Check sheet for the modelled part. Datum: model origin and axes. Units: mm. Face numbers are marked on the shaded views. Coordinates: 2 decimals unless noted, no trailing zeros. Write each loop counter-clockwise with the first axis right and the second up, starting at its lowest first coordinate (ties: lowest second). Pieces come first, ordered by that corner, then holes. Notation, with made-up numbers: (79, 84.5) - (87, 84.5) arc R14 cw to (87, 93.5) - close; hole circle Ø4 at (-25.5, 61.25). An arc over 180 degrees is marked (long way). Write each question's results on one line, items separated by ' | '.
from build123d import *

# Parameters (mm, degrees)
BOSS_EXTRUDE1_DEPTH = 12.7
CUT_EXTRUDE2_DEPTH  = 199.932436772
CUT_EXTRUDE1_DEPTH  = 104.050150898
CUT_EXTRUDE3_DEPTH  = 63.5
CHAMFER1_SIZE       = 1.5875
FILLET1_R           = 0.762
FILLET2_R           = 1.27


# Some blends are built 0.0001 mm under size
with BuildPart() as part:
    # Sketch1 → Boss-Extrude1 (new body)
    with BuildSketch(Plane(origin=(0, 0, 0), x_dir=(1, 0, 0), z_dir=(0, 1, 0))):
        with BuildLine():
            Line((-99.06, -12.7), (99.06, -12.7))
            Line((99.06, -12.7), (99.06, -11.1125))
            Line((99.06, -11.1125), (80.01, -11.1125))
            ThreePointArc((80.01, -11.1125), (75.519871939, -9.252628061), (73.66, -4.7625))
            Line((73.66, -4.7625), (73.66, 4.7625))
            ThreePointArc((73.66, 4.7625), (75.519871939, 9.252628061), (80.01, 11.1125))
            Line((80.01, 11.1125), (99.06, 11.1125))
            Line((99.06, 11.1125), (99.06, 12.7))
            Line((99.06, 12.7), (-99.06, 12.7))
            Line((-99.06, 12.7), (-99.06, 11.1125))
            Line((-99.06, 11.1125), (-80.01, 11.1125))
            ThreePointArc((-80.01, 11.1125), (-75.519871939, 9.252628061), (-73.66, 4.7625))
            Line((-73.66, 4.7625), (-73.66, -4.7625))
            ThreePointArc((-73.66, -4.7625), (-75.519871939, -9.252628061), (-80.01, -11.1125))
            Line((-80.01, -11.1125), (-99.06, -11.1125))
            Line((-99.06, -11.1125), (-99.06, -12.7))
        make_face()
    extrude(amount=BOSS_EXTRUDE1_DEPTH)

    # Sketch3 → Cut-Extrude2 (cut, through all)
    with BuildSketch(Plane.ZY.offset(99.06)):
        Polygon((11.1125, 12.7), (4.7625, 12.7), (-4.7625, 12.7), (-11.1125, 12.7), (-9.525, 6.35), (9.525, 6.35), align=None)
    extrude(amount=-CUT_EXTRUDE2_DEPTH, mode=Mode.SUBTRACT)

    # Sketch2 → Cut-Extrude1 (cut, through all)
    with BuildSketch(Plane.XY.offset(12.7)):
        Polygon((73.66, 12.7), (-73.66, 12.7), (-67.31, 6.35), (67.31, 6.35), align=None)
        with BuildLine():
            Line((97.263948776, 4.553948776), (92.71, 0))
            Line((92.71, 0), (99.06, 0))
            Line((99.06, 0), (99.06, 12.7))
            Line((99.06, 12.7), (92.71, 12.7))
            Line((92.71, 12.7), (97.263948776, 8.146051224))
            ThreePointArc((97.263948776, 8.146051224), (98.007897552, 6.35), (97.263948776, 4.553948776))
        make_face()
        with BuildLine():
            ThreePointArc((-97.263948776, 4.553948776), (-98.007897552, 6.35), (-97.263948776, 8.146051224))
            Line((-97.263948776, 8.146051224), (-92.71, 12.7))
            Line((-92.71, 12.7), (-99.06, 12.7))
            Line((-99.06, 12.7), (-99.06, 0))
            Line((-99.06, 0), (-92.71, 0))
            Line((-92.71, 0), (-97.263948776, 4.553948776))
        make_face()
    extrude(amount=-CUT_EXTRUDE1_DEPTH, mode=Mode.SUBTRACT)

    # Sketch4 → Revolve1 (revolve)
    with BuildSketch(Plane.ZY.offset(90.17)):
        with BuildLine():
            Line((12.7, 6.35), (12.7, 11.43))
            ThreePointArc((12.7, 11.43), (13.881381744, 9.01113492), (14.2875, 6.35))
            Line((14.2875, 6.35), (12.7, 6.35))
        make_face()
    revolve1 = revolve(axis=Axis((-90.17, 6.35, 0), (0, 0, 1)))

    # Mirror1: Revolve1 across plane
    add(revolve1.mirror(Plane.XY))

    # Sketch5 → Revolve2 (revolve)
    with BuildSketch(Plane(origin=(90.17, 0, 0), x_dir=(0, 0, -1), z_dir=(1, 0, 0))):
        with BuildLine():
            Line((11.1125, 6.35), (11.1125, 11.43))
            ThreePointArc((11.1125, 11.43), (9.931118256, 9.01113492), (9.525, 6.35))
            Line((9.525, 6.35), (11.1125, 6.35))
        make_face()
    revolve2 = revolve(axis=Axis((90.17, 6.35, 0), (0, 0, -1)))

    # Mirror2: Revolve2 across plane
    add(revolve2.mirror(Plane.XY))

    # Sketch6 → Cut-Extrude3 (cut, symmetric)
    with BuildSketch(Plane(origin=(0, 0, 0), x_dir=(0, 0, -1), z_dir=(1, 0, 0))):
        Polygon((-12.7, 0), (-11.1125, 0), (-12.7, 1.5875), align=None)
        Polygon((11.1125, 0), (12.7, 1.5875), (12.7, 0), align=None)
    extrude(amount=CUT_EXTRUDE3_DEPTH, both=True, mode=Mode.SUBTRACT)

    # Chamfer1
    chamfer1_edges = [part.edges().sort_by_distance(p)[0] for p in [
        (63.5, 0, 11.90625),
        (63.5, 0, -11.90625),
        (-63.5, 0, -11.90625),
        (-63.5, 0, 11.90625),
    ]]
    chamfer(chamfer1_edges, length=CHAMFER1_SIZE - 0.0001)  # a hair under: the kernel refuses the full size

    # Fillet1
    fillet1_edges = [part.edges().sort_by_distance(p)[0] for p in [
        (-98.007897552, 6.35, 12.7),
        (-92.71, 12.7, -11.90625),
        (-94.986974388, 10.423025612, -11.1125),
        (-94.986974388, 10.423025612, -12.7),
        (-94.986974388, 10.423025612, 11.1125),
        (-92.71, 12.7, 11.90625),
        (-94.986974388, 2.276974388, 12.7),
        (-98.007897552, 6.35, -11.1125),
        (-98.007897552, 6.35, 11.1125),
        (-94.986974388, 2.276974388, -11.1125),
        (-94.986974388, 2.276974388, 11.1125),
        (-98.007897552, 6.35, -12.7),
        (-94.986974388, 2.276974388, -12.7),
        (-94.986974388, 10.423025612, 12.7),
        (98.007897552, 6.35, 12.7),
        (92.71, 12.7, 11.90625),
        (92.71, 12.7, -11.90625),
        (94.986974388, 10.423025612, 12.7),
        (94.986974388, 2.276974388, 11.1125),
        (94.986974388, 2.276974388, -11.1125),
        (94.986974388, 2.276974388, -12.7),
        (98.007897552, 6.35, 11.1125),
        (94.986974388, 10.423025612, 11.1125),
        (94.986974388, 10.423025612, -11.1125),
        (98.007897552, 6.35, -12.7),
        (94.986974388, 10.423025612, -12.7),
        (94.986974388, 2.276974388, 12.7),
        (98.007897552, 6.35, -11.1125),
    ]]
    fillet(fillet1_edges, radius=FILLET1_R)

    # Fillet2
    # the kernel refuses this fillet: 1.27 mm, written as the material it takes off along each edge
    with BuildSketch(Plane(origin=(-75.90506403, 14.94506403, -12.7), x_dir=(-0.7071067811865446, -0.7071067811865505, 0), z_dir=(0.7071067811865506, -0.7071067811865446, 0))) as fillet2_piece_1_section:
        with BuildLine():
            CenterArc((FILLET2_R, -FILLET2_R), FILLET2_R, 90, 90)
            Line((0, -FILLET2_R), (0, 0))
            Line((0, 0), (FILLET2_R, 0))
        make_face()
    fillet2_piece_1 = extrude(amount=15.330256121, mode=Mode.PRIVATE)
    fillet2_piece_1 = split(fillet2_piece_1, bisect_by=Plane(origin=(-71.905795305, 6.35, -12.408746665), z_dir=(0, 1, 0)), keep=Keep.TOP, mode=Mode.PRIVATE)
    add(fillet2_piece_1, mode=Mode.SUBTRACT)
    with BuildSketch(Plane(origin=(-65.450815483, 4.490815483, -9.060203871), x_dir=(0.1230914909792504, -0.12309149097924957, -0.9847319278346824), z_dir=(-0.696310623822809, 0.6963106238228031, -0.17407765595558086))) as fillet2_piece_2_section:
        with BuildLine():
            CenterArc((FILLET2_R * 0.840960781889, FILLET2_R), FILLET2_R, 189.874961398, 80.125038602)
            Line((-FILLET2_R * 0.144223584254, FILLET2_R * 0.828501414858), (0, 0))
            Line((0, 0), (FILLET2_R * 0.840960781889, 0))
        make_face()
    fillet2_piece_2 = extrude(amount=14.459594166, mode=Mode.PRIVATE)
    fillet2_piece_2 = split(fillet2_piece_2, bisect_by=Plane(origin=(-71.646234354, 6.35, -10.770930609), z_dir=(0, 1, 0)), keep=Keep.TOP, mode=Mode.PRIVATE)
    add(fillet2_piece_2, mode=Mode.SUBTRACT)
    with BuildSketch(Plane(origin=(-75.519184517, 14.559184517, 11.577296129), x_dir=(-0.7177405625652845, -0.6755205294731655, -0.1688801323683837), z_dir=(0.69631062382278, -0.6963106238227741, -0.17407765595581334))) as fillet2_piece_3_section:
        with BuildLine():
            CenterArc((FILLET2_R * 0.840960781889, -FILLET2_R), FILLET2_R, 90, 80.125038602)
            Line((-FILLET2_R * 0.144223584254, -FILLET2_R * 0.828501414857), (0, 0))
            Line((0, 0), (FILLET2_R * 0.840960781889, 0))
        make_face()
    fillet2_piece_3 = extrude(amount=14.459594166, mode=Mode.PRIVATE)
    fillet2_piece_3 = split(fillet2_piece_3, bisect_by=Plane(origin=(-71.646234354, 6.35, 10.770930609), z_dir=(0, 1, 0)), keep=Keep.TOP, mode=Mode.PRIVATE)
    add(fillet2_piece_3, mode=Mode.SUBTRACT)
    with BuildSketch(Plane(origin=(-75.90506403, 14.94506403, 12.7), x_dir=(-0.7071067811865445, -0.7071067811865505, 0), z_dir=(0.7071067811865506, -0.7071067811865446, 0))) as fillet2_piece_4_section:
        with BuildLine():
            CenterArc((FILLET2_R, FILLET2_R), FILLET2_R, 180, 90)
            Line((0, FILLET2_R), (0, 0))
            Line((0, 0), (FILLET2_R, 0))
        make_face()
    fillet2_piece_4 = extrude(amount=15.330256121, mode=Mode.PRIVATE)
    fillet2_piece_4 = split(fillet2_piece_4, bisect_by=Plane(origin=(-71.905795305, 6.35, 12.408746665), z_dir=(0, 1, 0)), keep=Keep.TOP, mode=Mode.PRIVATE)
    add(fillet2_piece_4, mode=Mode.SUBTRACT)
    with BuildSketch(Plane(origin=(65.06493597, 4.10493597, -12.7), x_dir=(0.7071067811865445, -0.7071067811865506, 0), z_dir=(0.7071067811865506, 0.7071067811865445, 0))) as fillet2_piece_5_section:
        with BuildLine():
            CenterArc((FILLET2_R, -FILLET2_R), FILLET2_R, 90, 90)
            Line((0, -FILLET2_R), (0, 0))
            Line((0, 0), (FILLET2_R, 0))
        make_face()
    fillet2_piece_5 = extrude(amount=15.330256121, mode=Mode.PRIVATE)
    fillet2_piece_5 = split(fillet2_piece_5, bisect_by=Plane(origin=(71.905795305, 6.35, -12.408746665), z_dir=(0, 1, 0)), keep=Keep.TOP, mode=Mode.PRIVATE)
    add(fillet2_piece_5, mode=Mode.SUBTRACT)
    with BuildSketch(Plane(origin=(75.519184517, 14.559184517, -11.577296129), x_dir=(-0.12309149097927001, -0.12309149097926336, -0.9847319278346782), z_dir=(-0.6963106238228061, -0.6963106238228001, 0.17407765595560445))) as fillet2_piece_6_section:
        with BuildLine():
            CenterArc((FILLET2_R * 0.840960781889, FILLET2_R), FILLET2_R, 189.874961398, 80.125038602)
            Line((-FILLET2_R * 0.144223584254, FILLET2_R * 0.828501414858), (0, 0))
            Line((0, 0), (FILLET2_R * 0.84096078189, 0))
        make_face()
    fillet2_piece_6 = extrude(amount=14.459594166, mode=Mode.PRIVATE)
    fillet2_piece_6 = split(fillet2_piece_6, bisect_by=Plane(origin=(71.646234354, 6.35, -10.770930609), z_dir=(0, 1, 0)), keep=Keep.TOP, mode=Mode.PRIVATE)
    add(fillet2_piece_6, mode=Mode.SUBTRACT)
    with BuildSketch(Plane(origin=(65.06493597, 4.10493597, 12.7), x_dir=(0.7071067811865445, -0.7071067811865507, 0), z_dir=(0.7071067811865506, 0.7071067811865445, 0))) as fillet2_piece_7_section:
        with BuildLine():
            CenterArc((FILLET2_R, FILLET2_R), FILLET2_R, 180, 90)
            Line((0, FILLET2_R), (0, 0))
            Line((0, 0), (FILLET2_R, 0))
        make_face()
    fillet2_piece_7 = extrude(amount=15.330256121, mode=Mode.PRIVATE)
    fillet2_piece_7 = split(fillet2_piece_7, bisect_by=Plane(origin=(71.905795305, 6.35, 12.408746665), z_dir=(0, 1, 0)), keep=Keep.TOP, mode=Mode.PRIVATE)
    add(fillet2_piece_7, mode=Mode.SUBTRACT)
    with BuildSketch(Plane(origin=(65.450815483, 4.490815483, 9.060203871), x_dir=(0.7177405625652817, -0.6755205294731627, -0.16888013236840813), z_dir=(0.6963106238227829, 0.6963106238227769, 0.1740776559557897))) as fillet2_piece_8_section:
        with BuildLine():
            CenterArc((FILLET2_R * 0.840960781889, -FILLET2_R), FILLET2_R, 90, 80.125038602)
            Line((-FILLET2_R * 0.144223584254, -FILLET2_R * 0.828501414857), (0, 0))
            Line((0, 0), (FILLET2_R * 0.840960781889, 0))
        make_face()
    fillet2_piece_8 = extrude(amount=14.459594166, mode=Mode.PRIVATE)
    fillet2_piece_8 = split(fillet2_piece_8, bisect_by=Plane(origin=(71.646234354, 6.35, 10.770930609), z_dir=(0, 1, 0)), keep=Keep.TOP, mode=Mode.PRIVATE)
    add(fillet2_piece_8, mode=Mode.SUBTRACT)


solid = part.part
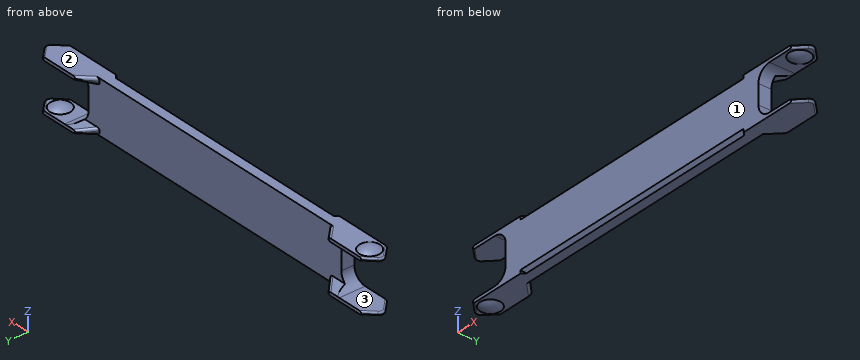
1. Material ranges on L1, parallel to Z at x = -31, y = 1.75; L2, parallel to X at y = 1.5, z = 0.5; L3, parallel to Z at x = -77, y = 11.25, recorded low to high. Write a range as [from, to].
Values follow:
L1: z = [-12.7, 12.7] | L2: x = [-73.66, 73.66] | L3: z = [-12.7, -10.75], [10.75, 12.7]
2. Sectioned sample at A-A (z = -0.5). Record the cut outline in (x, y), then the cut area to 3 significant figures.
Values follow:
outline: (-73.66, 0) - (73.66, 0) - (73.66, 6.35) - (-73.66, 6.35) - close | area: 935 mm^2
3. Go/stop test with flat-tipped pins: pin 1 (3 mm diameter, centred on y = 4.5, z = 0, fed in from -X); pin 2 (8 mm diameter, centred on x = 57.5, z = -1.5, fed in from +Y); pin 3 (4 mm diameter, centred on x = 22, y = 5.5, fed in from -Z); pin 4 (2 mm diameter, centred on x = -14, y = 8.5, fed in from -Z). Record where each tip stops, or that it passes through.
Values follow:
pin 1: stops at x = -73.66 | pin 2: stops at y = 6.35 | pin 3: stops at z = -12.7 | pin 4: passes through
4. Sectioned sample at B-B (x = -56). Record the cut outline in (y, z).
Values follow:
outline: (0, -11.11) - (1.59, -12.7) - (6.35, -12.7) - (6.35, 12.7) - (1.59, 12.7) - (0, 11.11) - close
5. Sectioned sample at C-C (z = 7). Record the cut outline in (x, y).
Values follow:
outline: (-74.07, 0) - (74.07, 0) - (74.07, 6.35) - (-74.07, 6.35) - close
6. Draft check along Z on the marked faces 1, 2 and 3. Enter one of: pulls with the +Z half, pulls with the -Z half, needs draft (parallel to the pull), parting line crosses it, or undercut.
Values follow:
face 1: needs draft | face 2: pulls with the +Z half | face 3: undercut
